For this review, take the finished solid that the model builds, in its own axes (mm). A direction names the side the tool comes from. Coordinates: 2 decimals unless noted, no trailing zeros. Write each loop counter-clockwise with the first axis right and the second up, starting at its lowest first coordinate (ties: lowest second). Pieces come first, ordered by that corner, then holes.
1) Mouldability with a two-part tool opening along Y and no side actions: class faces 1 (the face through (-38, 31, 13.97)), 2 (the face through (-34, -9.144, 7)), 3 (the face through (-5, -10.7, 6.9)) as pulls with the +Y half, pulls with the -Y half, needs draft (parallel to the pull), parting line crosses it, or undercut.
2) Insertion check: P1, Ø1.1, axis at x = -35, z = 5, coming from the +Y side; P2, Ø2, axis at x = -24.5, y = -0.5, coming from the +Z side; P3, Ø7, axis at y = 18.5, z = 7, coming from the +X side; P4, Ø1.5, axis at x = -22, z = 2, coming from the -Y side. Each pin has a flat end and moves straight along its axis. Give the tip position at first contact, or say it passes through.
3) To check wall thickness, follow line 1 along X through (y, z) = (-6, 6.75); line 2 along Y through (x, z) = (-2.5, 6); line 3 along Y through (x, z) = (-31, 2). State the ranges of each line that lie inside material, in increasing order.
4) We need section B-B on z = 4.75. Write out the cut boundary in (x, y), then the cut area to 3 significant figures.
5) We need section C-C on z = 10. Write out the cut boundary in (x, y).
6) We need section A-A on y = 7.5. Write out the cut boundary in (x, z), then the cut area to 3 significant figures.
7) For faces 4 (the face through (-19, 2.921, 5)), 5 (the face through (-36.322, -5, 7)), 6 (the face through (-36.322, 22, 2)), 7 (the face through (-2, 28.702, 8)), 8 (the face through (-8.89, 1, 11)), list the 3-axis set-ups (+Z, -Z, +X, -X, +Y, -Y) from which the entire face can be reached by the end or side of a thin tool; tool diameter is ignored.
8) We need section D-D on x = -34.5. Write out the cut boundary in (y, z).
from build123d import *

# Parameters (mm, degrees)
F0_W     = 10.795
F0_H     = 2.921
F1_DEPTH = 7.874
F2_DEPTH = 13.97
F0_W_2   = 3.048
F0_H_2   = 25.781
F3_DEPTH = 2.921
F0_H_3   = 3.937
F4_DEPTH = 13.97


with BuildPart() as f1:
    # F0 (on Top) → F1 (new body)
    with BuildSketch(Plane.XY):
        with Locations((-25.0825, 1.4605)):
            Rectangle(F0_W, F0_H)
        with Locations((-14.2875, 1.4605)):
            Rectangle(F0_W, F0_H)
    extrude(amount=F1_DEPTH)

    # F0 (on Top) → F2 (join)
    with BuildSketch(Plane.XY):
        Polygon((0, 2.921), (-3.048, 2.921), (-8.89, 2.921), (-8.89, 0), (-3.048, 0), (-3.048, -9.144), (-6.880294, -9.144), (-3.048, -12.319), (0, -12.319), (0, -9.144), align=None)
        Polygon((-30.48, 0), (-30.48, 2.921), (-36.322, 2.921), (-39.37, 2.921), (-39.37, -9.144), (-39.37, -12.319), (-36.322, -12.319), (-32.489706, -9.144), (-36.322, -9.144), (-36.322, 0), align=None)
    extrude(amount=F2_DEPTH)

    # F0 (on Top) → F3 (join)
    with BuildSketch(Plane.XY):
        with Locations((-1.524, 15.8115)):
            Rectangle(F0_W_2, F0_H_2)
        with Locations((-37.846, 15.8115)):
            Rectangle(F0_W_2, F0_H_2)
    extrude(amount=F3_DEPTH)

    # F0 (on Top) → F4 (join)
    with BuildSketch(Plane.XY):
        with Locations((-1.524, 30.6705)):
            Rectangle(F0_W_2, F0_H_3)
        with Locations((-37.846, 30.6705)):
            Rectangle(F0_W_2, F0_H_3)
    extrude(amount=F4_DEPTH)


solid = f1.part
Result:
1. face 1: needs draft
1. face 2: undercut
1. face 3: pulls with the -Y half
2. P1: stops at y = 2.92
2. P2: stops at z = 7.87
2. P3: passes through
2. P4: stops at y = 0
3. line 1: x = -39.37 to -36.32, -3.05 to 0
3. line 2: y = -12.32 to 2.92, 28.7 to 32.64
3. line 3: y = 0 to 2.92
4. outline: (-39.37, -12.32) - (-36.32, -12.32) - (-32.49, -9.14) - (-36.32, -9.14) - (-36.32, 0) - (-3.05, 0) - (-3.05, -9.14) - (-6.88, -9.14) - (-3.05, -12.32) - (0, -12.32) - (0, 2.92) - (-39.37, 2.92) - close; (-39.37, 28.7) - (-36.32, 28.7) - (-36.32, 32.64) - (-39.37, 32.64) - close; (-3.05, 28.7) - (0, 28.7) - (0, 32.64) - (-3.05, 32.64) - close
4. area: 226 mm2
5. outline: (-39.37, -12.32) - (-36.32, -12.32) - (-32.49, -9.14) - (-36.32, -9.14) - (-36.32, 0) - (-30.48, 0) - (-30.48, 2.92) - (-39.37, 2.92) - close; (-39.37, 28.7) - (-36.32, 28.7) - (-36.32, 32.64) - (-39.37, 32.64) - close; (-8.89, 0) - (-3.05, 0) - (-3.05, -9.14) - (-6.88, -9.14) - (-3.05, -12.32) - (0, -12.32) - (0, 2.92) - (-8.89, 2.92) - close; (-3.05, 28.7) - (0, 28.7) - (0, 32.64) - (-3.05, 32.64) - close
6. outline: (-39.37, 0) - (-36.32, 0) - (-36.32, 2.92) - (-39.37, 2.92) - close; (-3.05, 0) - (0, 0) - (0, 2.92) - (-3.05, 2.92) - close
6. area: 17.8 mm2
7. face 4: +Z
7. face 5: +Z, -Z
7. face 6: +Z, -Z, +Y
7. face 7: +Z, +X, -X
7. face 8: +Z, +Y, -Y
8. outline: (-10.81, 0) - (-9.14, 0) - (-9.14, 13.97) - (-10.81, 13.97) - close; (0, 0) - (2.92, 0) - (2.92, 13.97) - (0, 13.97) - close
